For this review, take the finished solid that the model builds, in its own axes (mm). Face numbers are marked on the shaded views. Round coordinates to 2 decimals unless told otherwise and drop trailing zeros. Write each loop counter-clockwise with the first axis right and the second up, starting at its lowest first coordinate (ties: lowest second). Pieces come first, ordered by that corner, then holes. Notation, with made-up numbers: M 26,87.25 L 73,87.25 A19 ccw 73,105.25 Z; hole C 77,-17 d2. An arc over 180 degrees is marked long. Write each question's results on one line, items separated by ' | '. Start each with the question number.
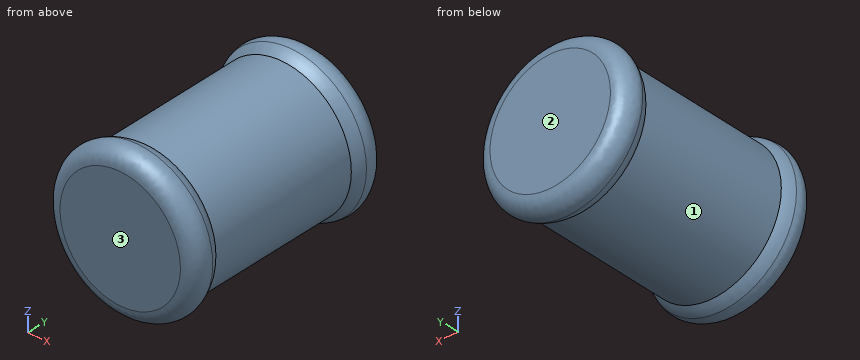
```python
from build123d import *

# Parameters (mm, degrees)
F0_R     = 2.25
F1_DEPTH = 5
F2_R     = 2.5
F2_R_2   = 2.25
F3_DEPTH = 1
F5_R     = 0.5
F6_R     = 2.5
F6_R_2   = 2.25
F7_DEPTH = 1
F9_R     = 0.5


# Not quite as in the source:
# - a fillet or chamfer that OpenCascade refuses, or shapes differently, is made with other operations: its cross-section is extruded or revolved along the edge and cut away or added


with BuildPart() as f1:
    # F0 (on Front) → F1 (new body)
    with BuildSketch(Plane.XZ):
        Circle(F0_R)
    extrude(amount=F1_DEPTH)

    # F2 (on face) → F3 (join)
    with BuildSketch(Plane.XZ.offset(5)):
        Circle(F2_R)
        Circle(F2_R_2, mode=Mode.SUBTRACT)
        Circle(F2_R_2)
    extrude(amount=F3_DEPTH)

    # F4: fillet of radius 1 on 1 edges, made by hand

    # F4_s1 → F4_t2 (revolve, cut)
    with BuildSketch(Plane.XY):
        with BuildLine():
            ThreePointArc((2.5, -5.6614378278), (2.4354143467, -5.3078844372), (2.25, -5))
            Line((2.25, -5), (2.5, -5))
            Line((2.5, -5), (2.5, -5.6614378278))
        make_face()
    revolve(axis=Axis((0, -5, 0), (0, -1, 0)), mode=Mode.SUBTRACT)

    # F5
    f5_edges = [f1.edges().sort_by_distance(p)[0] for p in [
        (-2.5, -6, 0),
    ]]
    fillet(f5_edges, radius=F5_R)

    # F6 (on face) → F7 (join)
    with BuildSketch(Plane(origin=(0, 0, 0), x_dir=(-1, 0, 0), z_dir=(0, 1, 0))):
        Circle(F6_R)
        Circle(F6_R_2, mode=Mode.SUBTRACT)
        Circle(F6_R_2)
    extrude(amount=F7_DEPTH)

    # F8: fillet of radius 1 on 1 edges, made by hand

    # F8_s1 → F8_t2 (revolve, cut)
    with BuildSketch(Plane.XY):
        with BuildLine():
            ThreePointArc((-2.5, 0.6614378278), (-2.4354143467, 0.3078844372), (-2.25, 0))
            Line((-2.25, 0), (-2.5, 0))
            Line((-2.5, 0), (-2.5, 0.6614378278))
        make_face()
    revolve(axis=Axis((0, 0, 0), (0, 1, 0)), mode=Mode.SUBTRACT)

    # F9
    f9_edges = [f1.edges().sort_by_distance(p)[0] for p in [
        (2.5, 1, 0),
    ]]
    fillet(f9_edges, radius=F9_R)


solid = f1.part
```
Item 1: Mouldability with a two-part tool opening along Y and no side actions: class the marked faces 1, 2 and 3 as pulls with the +Y half, pulls with the -Y half, needs draft (parallel to the pull), parting line crosses it, or undercut.
Item 2: Insertion check: P1, Ø1, axis at y = -0.5, z = 1.5, coming from the -X side. The pin has a flat end and moves straight along its axis. Give the tip position at first contact, or say it passes through.
Item 3: For probe 1 along X at (y, z) = (-4.5, -0.05); probe 2 along Y at (x, z) = (0.1, -2.2); probe 3 along Z at (x, y) = (1.75, 0.5), list the stretches that pass through material, from the lowest coordinate up.
Item 4: We need section A-A on y = -3.5. State the section outline as (x, z) points.
Numbers:
1) face 1: undercut | face 2: pulls with the +Y half | face 3: pulls with the -Y half
2) P1: stops at x = -2.02
3) probe 1: x = -2.25 to 2.25 | probe 2: y = -5.94 to 0.94 | probe 3: z = -1.75 to 1.75
4) outline: C 0,0 d4.5
